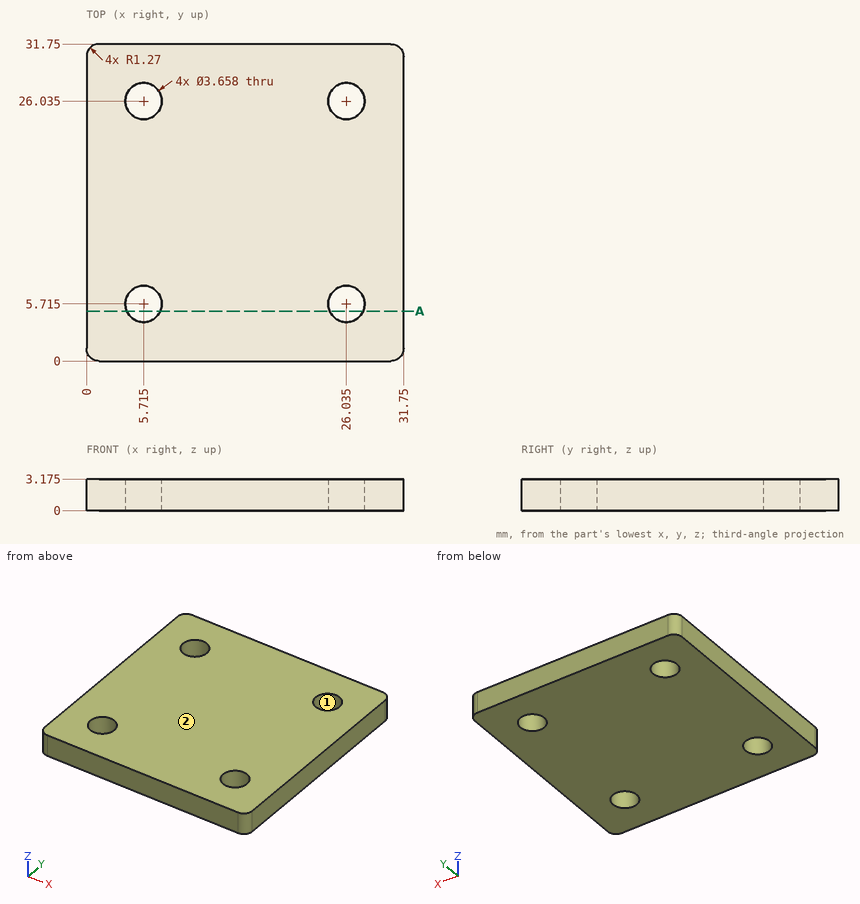
Print and shaded views of the part. All mm, measured from the part's lowest x, y and z. Round coordinates to 2 decimals unless told otherwise and drop trailing zeros. Return JSON: item names as keys, results as strings. Group by question number.
Q1. Pin check, flat tip, straight feed: pin 1 (6 mm diameter, centred on x = 26.035, y = 5.715, fed in from +Z) (3 decimals). Stop position of the tip, or through.
Q2. Mould opens along X. For the marked faces 1 and 2 say: pulls with the +X half, pulls with the -X half, needs draft (parallel to the pull), parting line crosses it, or undercut.
Q3. Probe L1, parallel to X at y = 4.5, z = 1.8; L2, parallel to Y at x = 5, z = 0.25. List the from-to ranges inside material, lowest first. Write a range as [from, to].
Q4. Saw through at A-A on y = 5. State how many separate pieces and enclosed holes the cut face has.
Answer:
{
 "1": {"pin 1": "z = 3.175"},
 "2": {"face 1": "undercut", "face 2": "needs draft"},
 "3": {"L1": "[0, 4.35], [7.08, 24.67], [27.4, 31.75]", "L2": "[0, 4.03], [7.4, 24.35], [27.72, 31.75]"},
 "4": {"separate pieces": "3", "enclosed holes": "0"}
}
